Source: three-view drawing plus pictorial views. Frame: mm from the lowest corner of the part. Give positions to 0.01 mm unless a question says otherwise; leave off trailing zeros. Loops run counter-clockwise (first coordinate to the right, second up) from the corner with the lowest first, then second, coordinate; pieces in that order, holes last. Notation, with made-up numbers: (-21.75, 83) - (10.25, 83) arc R20 cw to (10.25, 103) - close; hole circle Ø4 at (34.25, 84.5). An arc over 180 degrees is marked (long way). Put each result on its own line as item: value.
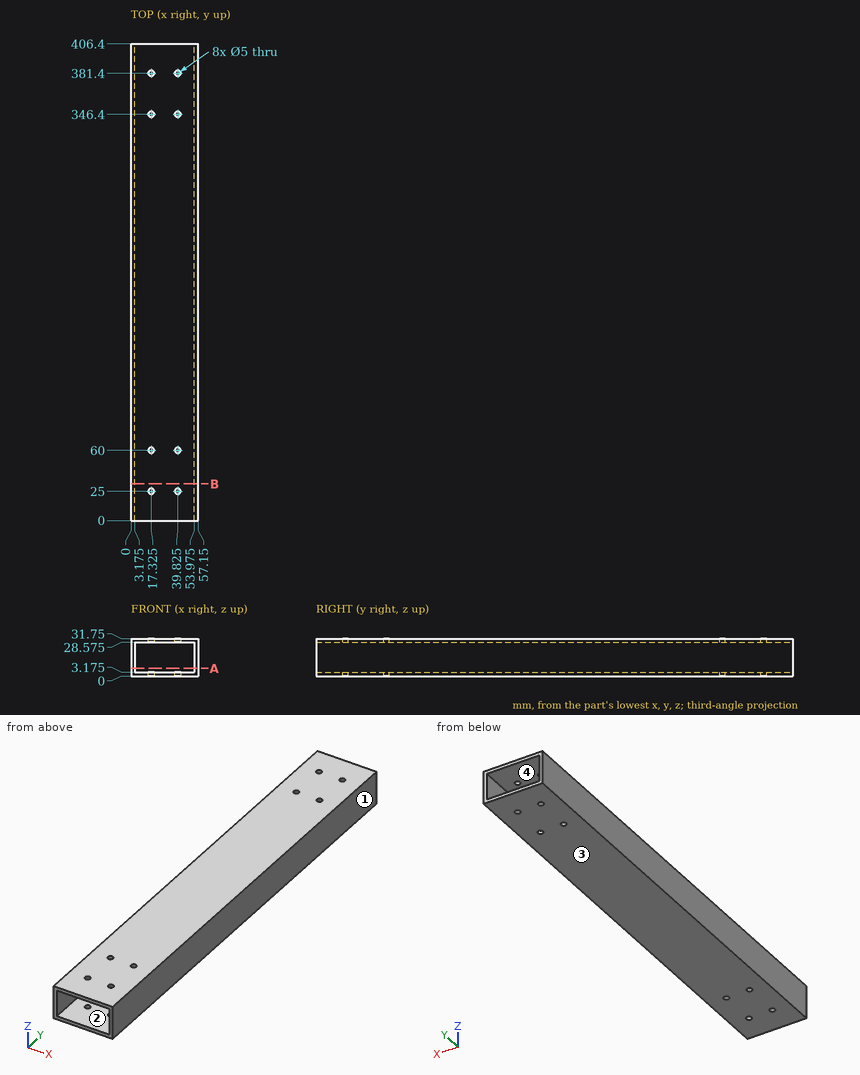
1) Mould query, pull axis Z, two halves, no side actions, for the marked faces 1, 2, 3 and 4. Classes: pulls with the +Z half, pulls with the -Z half, needs draft (parallel to the pull), parting line crosses it, or undercut.
Check result:
face 1: needs draft
face 2: undercut
face 3: pulls with the -Z half
face 4: undercut
2) Section query B-B, the plane y = 31.5. Output: boundary loops of the cut face in (x, z) (3 decimals), plus the area to 3 significant figures.
Check result:
outline: (0, 0) - (57.15, 0) - (57.15, 31.75) - (0, 31.75) - close; hole (3.175, 3.175) - (53.975, 3.175) - (53.975, 28.575) - (3.175, 28.575) - close
area: 524 mm²
3) Section query A-A, the plane z = 6.5. Output: boundary loops of the cut face in (x, y) (3 decimals), plus the area to 3 significant figures.
Check result:
outline: (0, 0) - (3.175, 0) - (3.175, 406.4) - (0, 406.4) - close; (53.975, 0) - (57.15, 0) - (57.15, 406.4) - (53.975, 406.4) - close
area: 2,580 mm²
4) Pin query (flat end, axial travel): P1, Ø4.5, axis at x = 17.325, y = 60, coming from the +Z side. Return the tip coordinate at first contact, or that it passes through.
Check result:
P1: through
5) Material intervals for line 1 along X through (y, z) = (346, 1); line 2 along X through (y, z) = (346.4, 0.95) (3 decimals); line 3 along Z through (x, y) = (49, 360) (3 decimals), sorted ascending. Write a range as [from, to].
Check result:
line 1: [0, 14.86], [19.79, 37.36], [42.29, 57.15]
line 2: [0, 14.825], [19.825, 37.325], [42.325, 57.15]
line 3: [0, 3.175], [28.575, 31.75]
